Work out the finished part from the listing and answer in its coordinate system (mm). A direction names the side the tool comes from. Coordinates: 2 decimals unless noted, no trailing zeros. Order: outer loops, then holes, each group sorted by start corner. A loop starts at its lowest first (then second) coordinate and runs counter-clockwise, first axis right, second up. Notation, with made-up numbers: M -3.75,87 L 20.25,87 A31 ccw 20.25,112 Z; hole C 26,77 d1. An arc over 180 degrees is marked long. Use a Markdown table: item, result.
from build123d import *

# Parameters (mm, degrees)
SKETCH1_R           = 2.5
BOSS_EXTRUDE1_DEPTH = 10
SKETCH2_W           = 20
SKETCH2_H           = 20
BOSS_EXTRUDE2_DEPTH = 25
FILLET1_R           = 7


with BuildPart() as part:
    # Sketch1 → Boss-Extrude1 (new body)
    with BuildSketch(Plane.XY):
        Circle(SKETCH1_R)
    extrude(amount=BOSS_EXTRUDE1_DEPTH)

    # Sketch2 → Boss-Extrude2 (add)
    with BuildSketch(Plane.XY.offset(10)):
        Rectangle(SKETCH2_W, SKETCH2_H)
    extrude(amount=BOSS_EXTRUDE2_DEPTH)

    # Fillet1
    fillet1_edges = [part.edges().sort_by_distance(p)[0] for p in [
        (10, -10, 22.5),
        (10, 10, 22.5),
        (-10, 10, 22.5),
        (-10, -10, 22.5),
    ]]
    fillet(fillet1_edges, radius=FILLET1_R)


solid = part.part
1. Find the intervals of material crossed by probe 1 along Z at (x, y) = (2.75, -4.5); probe 2 along X at (y, z) = (-1, 7); probe 3 along Y at (x, z) = (-8.75, 30), in increasing order.
Answers below:
| item | result |
|---|---|
| probe 1 | 10 to 35 |
| probe 2 | -2.29 to 2.29 |
| probe 3 | -6.99 to 6.99 |
2. Section C-C on x = 7.75 is taken. Determine the outline of the cut face in (y, z), then the cut area to 3 significant figures.
Answers below:
| item | result |
|---|---|
| outline | M -8.14,10 L 8.14,10 L 8.14,35 L -8.14,35 Z |
| area | 407 mm² |
3. Flat-ended cylindrical pins translate along their axes: P1, Ø10, axis at x = 4, y = 7, coming from the -Z side; P2, Ø5, axis at y = 6, z = 28.5, coming from the -X side. Find the tip coordinate at first contact, or state that the pin passes through.
Answers below:
| item | result |
|---|---|
| P1 | z = 10 |
| P2 | x = -9.98 |
4. Section B-B on z = 12 is taken. Determine the outline of the cut face in (x, y), then the cut area to 3 significant figures.
Answers below:
| item | result |
|---|---|
| outline | M -10,-3 A7 ccw -3,-10 L 3,-10 A7 ccw 10,-3 L 10,3 A7 ccw 3,10 L -3,10 A7 ccw -10,3 Z |
| area | 358 mm² |
5. Section D-D on z = 7.5 is taken. Determine the outline of the cut face in (x, y), then the cut area to 3 significant figures.
Answers below:
| item | result |
|---|---|
| outline | C 0,0 d5 |
| area | 19.6 mm² |
6. Section A-A on y = 0 is taken. Determine the outline of the cut face in (x, z), then the cut area to 3 significant figures.
Answers below:
| item | result |
|---|---|
| outline | M -10,10 L -2.5,10 L -2.5,0 L 2.5,0 L 2.5,10 L 10,10 L 10,35 L -10,35 Z |
| area | 550 mm² |
7. For faces 1 (the face through (-0.54, -2.44, 4.93)), 2 (the face through (0, 0, 0)), determine the directions among +Z, -Z, +X, -X, +Y, -Y from which every point of the face is accessible in a straight line to the end or side of a thin tool.
Answers below:
| item | result |
|---|---|
| face 1 | -Z |
| face 2 | -Z, +X, -X, +Y, -Y |
